For this review, use the dimensioned drawing (mm, ordinates from the lowest corner) and the shaded views. Coordinates: 2 decimals unless noted, no trailing zeros. Loops run counter-clockwise (first coordinate to the right, second up) from the corner with the lowest first, then second, coordinate; pieces in that order, holes last. Notation, with made-up numbers: (25.5, 53.25) - (32.5, 53.25) arc R33 ccw to (32.5, 88.25) - close; hole circle Ø4 at (3.5, 39). An arc over 180 degrees is marked (long way). Use a Markdown table: item, result. Add a question column.
1) Add section A-A, the plane z = 78.5. Give the boundary of the cut face in (x, y), and give its area (3 significant figures).
2) To check wall thickness, follow L1, parallel to X at y = 6, z = 43; L2, parallel to Z at x = 11.5, y = 9; L3, parallel to Z at x = 84.5, y = 6.5. State the ranges of each line that lie inside material, in increasing order. Write a range as [from, to].
3) Add section B-B, the plane y = 8.25. Give the boundary of the cut face in (x, z), and give its area (3 significant figures).
4) Clearance check with flat-ended pins moving along their axes: pin 1 (6 mm diameter, centred on x = 78, y = 8.5, fed in from -Z); pin 2 (6 mm diameter, centred on x = 24.5, y = 9, fed in from +Z); pin 3 (1.5 mm diameter, centred on y = 7.5, z = 41.5, fed in from +X); pin 4 (12 mm diameter, centred on x = 19, z = 47.5, fed in from -Y). State where each tip first meets the part, or that it passes through.
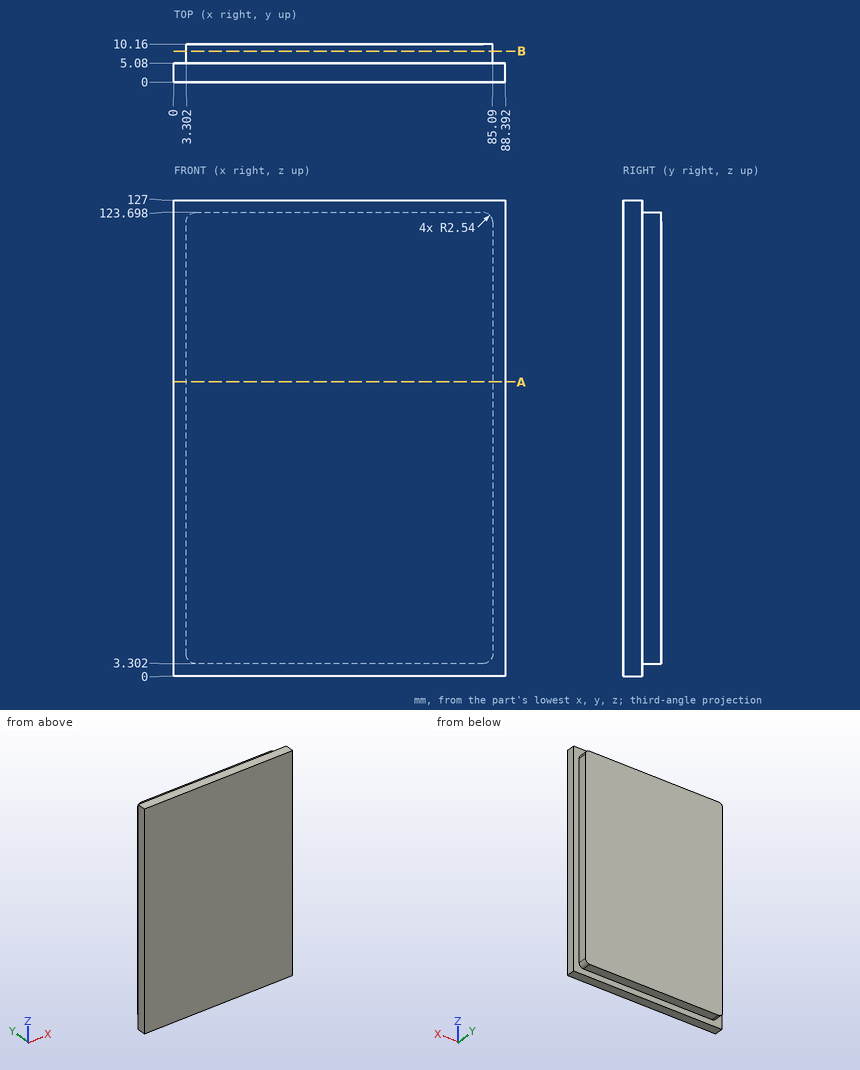
From the geometry:
| question | item | result |
|---|---|---|
| 1 | outline | (0, 0) - (88.39, 0) - (88.39, 5.08) - (85.09, 5.08) - (85.09, 10.16) - (3.3, 10.16) - (3.3, 5.08) - (0, 5.08) - close |
| 1 | area | 865 mm^2 |
| 2 | L1 | x = [3.3, 85.09] |
| 2 | L2 | z = [3.3, 123.7] |
| 2 | L3 | z = [4.21, 122.79] |
| 3 | outline | (3.3, 5.84) arc R2.54 ccw to (5.84, 3.3) - (82.55, 3.3) arc R2.54 ccw to (85.09, 5.84) - (85.09, 121.16) arc R2.54 ccw to (82.55, 123.7) - (5.84, 123.7) arc R2.54 ccw to (3.3, 121.16) - close |
| 3 | area | 9,840 mm^2 |
| 4 | pin 1 | stops at z = 3.3 |
| 4 | pin 2 | stops at z = 123.7 |
| 4 | pin 3 | stops at x = 85.09 |
| 4 | pin 4 | stops at y = 0 |
